Source: CAD feature listing. Evaluate the final solid. Frame: model axes, mm. Give positions to 0.01 mm unless a question says otherwise; leave off trailing zeros. Loops run counter-clockwise (first coordinate to the right, second up) from the corner with the lowest first, then second, coordinate; pieces in that order, holes last.
from build123d import *

# Parameters (mm, degrees)
SKETCH1_W           = 10
SKETCH1_H           = 10
BOSS_EXTRUDE1_DEPTH = 800
SKETCH4_R           = 2.5
BOSS_EXTRUDE3_DEPTH = 10


with BuildPart() as part:
    # Sketch1 → Boss-Extrude1 (new body)
    with BuildSketch(Plane.XY):
        Rectangle(SKETCH1_W, SKETCH1_H)
    extrude(amount=BOSS_EXTRUDE1_DEPTH)

    # Sketch4 → Boss-Extrude3 (add)
    with BuildSketch(Plane.ZY.offset(5)):
        with Locations(Location((10, 0, 0), (0, 0, 180))):
            Circle(SKETCH4_R)
        with Locations(Location((790, 0, 0), (0, 0, 180))):
            Circle(SKETCH4_R)
    extrude(amount=BOSS_EXTRUDE3_DEPTH)


solid = part.part
1) Ray query, probe 1 along Z at (x, y) = (-5.25, 0.75); probe 2 along X at (y, z) = (3.75, 147.5); probe 3 along Z at (x, y) = (-5.75, 2). Return the intervals inside material, ascending.
Checks:
probe 1: z = 7.62 to 12.38, 787.62 to 792.38
probe 2: x = -5 to 5
probe 3: z = 8.5 to 11.5, 788.5 to 791.5
2) Cut plane A-A (y = 0). Return loops of the section in (x, z), and give its area (3 significant figures).
Checks:
outline: (-15, 7.5) - (-5, 7.5) - (-5, 0) - (5, 0) - (5, 800) - (-5, 800) - (-5, 792.5) - (-15, 792.5) - (-15, 787.5) - (-5, 787.5) - (-5, 12.5) - (-15, 12.5) - close
area: 8,100 mm2
3) Contact query for flat-ended pins moving along their axis: P1, Ø3, axis at x = -10.5, y = 0.5, coming from the -Z side; P2, Ø5, axis at y = 1, z = 133.5, coming from the -X side; P3, Ø12, axis at x = -11.5, z = 365.5, coming from the -Y side. Output: stop coordinate, or through.
Checks:
P1: stops at z = 7.5
P2: stops at x = -5
P3: passes through
4) Cut plane B-B (z = 131). Return loops of the section in (x, y), and give its area (3 significant figures).
Checks:
outline: (-5, -5) - (5, -5) - (5, 5) - (-5, 5) - close
area: 100 mm2
